Job drawing, mm, ordinate dimensions from the low corner. One solid piece. A direction names the side the tool comes from. Coordinates: 2 decimals unless noted, no trailing zeros. Loops run counter-clockwise (first coordinate to the right, second up) from the corner with the lowest first, then second, coordinate; pieces in that order, holes last. Notation, with made-up numbers: (-40, 3) -> (3, 3) arc R12 cw to (3, 20) -> close; hole circle Ø1 at (21, 37). An arc over 180 degrees is marked (long way). Use one line per item in the form item = value. Start each with the question number.
(1) Pin check, flat tips, straight feed: P1, Ø2, axis at y = 6.5, z = 10.5, coming from the +X side; P2, Ø4, axis at x = 7, y = 10.5, coming from the +Z side; P3, Ø12, axis at x = 39, z = 15, coming from the +Y side. Stop position of each tip, or through.
(2) Band-saw the part on C-C on y = 4.5. Give the cut face in (x, z).
(3) Band-saw the part on D-D on z = 1.75. Give the cut face in (x, y).
(4) 3-axis set-ups, long thin cutter, end or side, ignore diameter. For the marked faces 5 and 6: which of +Z, -Z, +X, -X, +Y, -Y reach the whole face in a straight line?
(5) Band-saw the part on B-B on x = 12. Give the cut face in (y, z), then the cut area to 3 significant figures.
(6) Mould opens along Y. For the marked faces 1, 2, 3 and 4 say: +Y half, -Y half, draft (parallel to the pull), parting line (faces both ways), or undercut.
(7) Band-saw the part on A-A on z = 12. Give the cut face in (x, y), then the cut area to 3 significant figures.
(8) Drill centre lines: L1, parallel to X at y = 3.95, z = 12; L2, parallel to Z at x = 12, y = 1.9; L3, parallel to Y at x = 13.25, z = 3.9. Where is each one in solid material? Low to high. Write a range as [from, to].
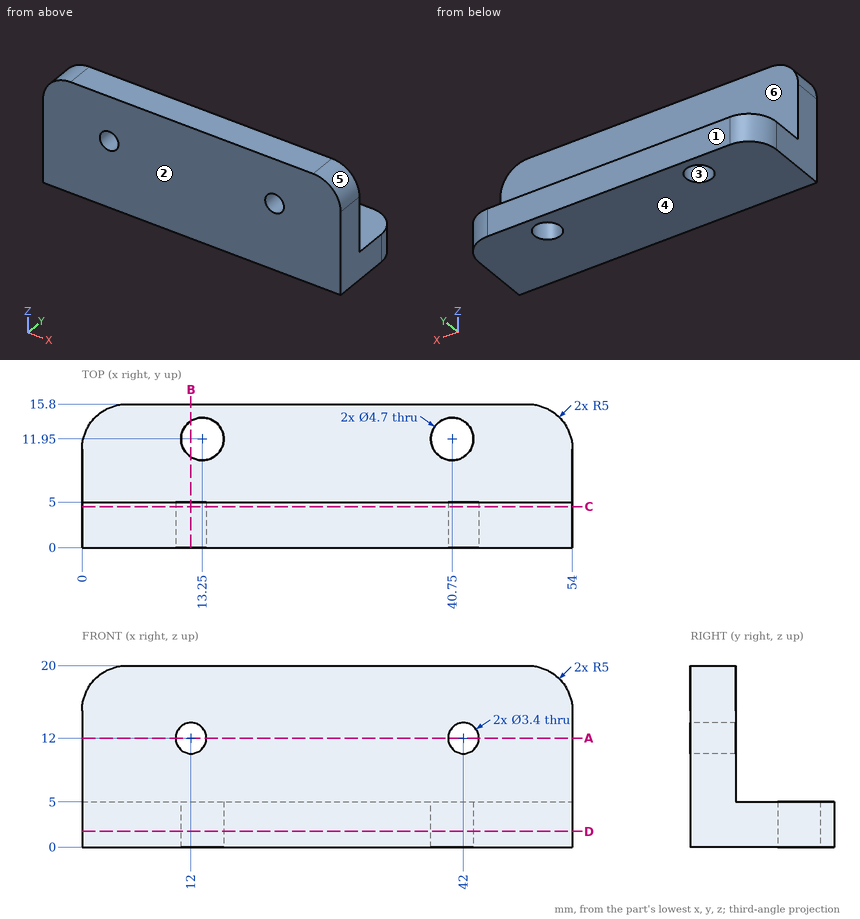
A:
q1.P1 = through
q1.P2 = 5
q1.P3 = 5
q2.outline = (0, 0) -> (54, 0) -> (54, 15) arc R5 ccw to (49, 20) -> (5, 20) arc R5 ccw to (0, 15) -> close; hole circle Ø3.4 at (12, 12); hole circle Ø3.4 at (42, 12)
q3.outline = (0, 0) -> (54, 0) -> (54, 10.8) arc R5 ccw to (49, 15.8) -> (5, 15.8) arc R5 ccw to (0, 10.8) -> close; hole circle Ø4.7 at (13.25, 11.95); hole circle Ø4.7 at (40.75, 11.95)
q4.face_5 = +Z, +X, +Y, -Y
q4.face_6 = +Z, +X, -X, +Y
q5.outline = (0, 0) -> (9.96, 0) -> (9.96, 5) -> (5, 5) -> (5, 10.3) -> (0, 10.3) -> close; (0, 13.7) -> (5, 13.7) -> (5, 20) -> (0, 20) -> close; (13.94, 0) -> (15.8, 0) -> (15.8, 5) -> (13.94, 5) -> close
q5.area = 117 mm²
q6.face_1 = +Y half
q6.face_2 = -Y half
q6.face_3 = undercut
q6.face_4 = draft
q7.outline = (0, 0) -> (10.3, 0) -> (10.3, 5) -> (0, 5) -> close; (13.7, 0) -> (40.3, 0) -> (40.3, 5) -> (13.7, 5) -> close; (43.7, 0) -> (54, 0) -> (54, 5) -> (43.7, 5) -> close
q7.area = 236 mm²
q8.L1 = [0, 10.3], [13.7, 40.3], [43.7, 54]
q8.L2 = [0, 10.3], [13.7, 20]
q8.L3 = [0, 9.6], [14.3, 15.8]
